```python
from build123d import *

# Parameters (mm, degrees)
SKETCH1_W           = 175
SKETCH1_H           = 77
SKETCH1_W_2         = 170
SKETCH1_H_2         = 69
BOSS_EXTRUDE1_DEPTH = 105
SKETCH2_W           = 175
SKETCH2_H           = 77
BOSS_EXTRUDE2_DEPTH = 3
SKETCH3_W           = 70
SKETCH3_H           = 80
SKETCH3_W_2         = 43
SKETCH3_H_2         = 62
CUT_EXTRUDE1_DEPTH  = 2.5
SKETCH4_W           = 12
SKETCH4_H           = 3
SKETCH4_W_2         = 24.903681778
SKETCH4_H_2         = 5
SKETCH4_W_3         = 25
SKETCH4_R           = 3
CUT_EXTRUDE2_DEPTH  = 12.5
SKETCH5_W           = 17.65
SKETCH5_H           = 18.35
CUT_EXTRUDE3_DEPTH  = 10
SKETCH6_W           = 5
SKETCH6_H           = 5
CUT_EXTRUDE4_DEPTH  = 10


with BuildPart() as part:
    # Sketch1 → Boss-Extrude1 (new body)
    with BuildSketch(Plane(origin=(0, 0, 0), x_dir=(1, 0, 0), z_dir=(0, 1, 0))):
        with Locations((-14.5, -36.5)):
            Rectangle(SKETCH1_W, SKETCH1_H)
        with Locations((-15, -35.5)):
            Rectangle(SKETCH1_W_2, SKETCH1_H_2, mode=Mode.SUBTRACT)
    extrude(amount=BOSS_EXTRUDE1_DEPTH)

    # Sketch2 → Boss-Extrude2 (add)
    with BuildSketch(Plane(origin=(0, 0, 0), x_dir=(-1, 0, 0), z_dir=(0, -1, 0))):
        with Locations((14.5, -36.5)):
            Rectangle(SKETCH2_W, SKETCH2_H)
    extrude(amount=-BOSS_EXTRUDE2_DEPTH)

    # Sketch3 → Cut-Extrude1 (cut)
    with BuildSketch(Plane.XY.offset(75)):
        with Locations((31, 57)):
            Rectangle(SKETCH3_W, SKETCH3_H)
        with Locations((-73.5, 66)):
            Rectangle(SKETCH3_W_2, SKETCH3_H_2)
    extrude(amount=-CUT_EXTRUDE1_DEPTH, mode=Mode.SUBTRACT)

    # Sketch4 → Cut-Extrude2 (cut)
    with BuildSketch(Plane.XY.offset(75)):
        with Locations((-28, 88.5)):
            Rectangle(SKETCH4_W, SKETCH4_H)
        with Locations((-73.5, 32.5)):
            Rectangle(SKETCH4_W_2, SKETCH4_H_2)
        with Locations((31, 14.5)):
            Rectangle(SKETCH4_W_3, SKETCH4_H_2)
        with Locations((-28, 51)):
            Circle(SKETCH4_R)
    extrude(amount=-CUT_EXTRUDE2_DEPTH, mode=Mode.SUBTRACT)

    # Sketch5 → Cut-Extrude3 (cut)
    with BuildSketch(Plane.XY.offset(1)):
        with Locations((48.75, 12.175)):
            Rectangle(SKETCH5_W, SKETCH5_H)
    extrude(amount=-CUT_EXTRUDE3_DEPTH, mode=Mode.SUBTRACT)

    # Sketch6 → Cut-Extrude4 (cut)
    with BuildSketch(Plane.ZY.offset(-70)):
        with Locations((35.5, 5.5)):
            Rectangle(SKETCH6_W, SKETCH6_H)
    extrude(amount=-CUT_EXTRUDE4_DEPTH, mode=Mode.SUBTRACT)


solid = part.part
```
CAD build for the part. Positions are in the model's coordinates, mm. A direction names the side the tool comes from. Coordinates: 2 decimals unless noted, no trailing zeros. Order: outer loops, then holes, each group sorted by start corner. A loop starts at its lowest first (then second) coordinate and runs counter-clockwise, first axis right, second up. Notation, with made-up numbers: (-8.5, 68.25) - (34.5, 68.25) arc R18 cw to (34.5, 100.25) - close; hole circle Ø2 at (43.25, -26). An arc over 180 degrees is marked (long way). Answer in a Markdown table with one row per item.
1. Drill centre lines: L1, parallel to Y at x = -28, z = 73.25; L2, parallel to Z at x = 40.5, y = 51; L3, parallel to X at y = 15, z = 70.5. Where is each one in solid material? Low to high. Write a range as from..to.
Answer:
| item | result |
|---|---|
| L1 | 0..48, 54..87, 90..105 |
| L2 | -2..1, 70..72.5 |
| L3 | -102..18.5, 43.5..73 |
2. Slice it at A-A, the plane y = 14. List the corners of the cut face in (x, z) (3 decimals).
Answer:
| item | result |
|---|---|
| outline | (-102, -2) - (39.925, -2) - (39.925, 1) - (-100, 1) - (-100, 70) - (18.5, 70) - (18.5, 75) - (-102, 75) - close; (43.5, 70) - (70, 70) - (70, 1) - (57.575, 1) - (57.575, -2) - (73, -2) - (73, 75) - (43.5, 75) - close |
3. Slice it at D-D, the plane x = -28. List the corners of the cut face in (y, z).
Answer:
| item | result |
|---|---|
| outline | (0, -2) - (105, -2) - (105, 1) - (3, 1) - (3, 70) - (48, 70) - (48, 75) - (0, 75) - close; (54, 70) - (87, 70) - (87, 75) - (54, 75) - close; (90, 70) - (105, 70) - (105, 75) - (90, 75) - close |
4. Pull direction Z, two halves, no side cores. Call faces 4 (the face through (-16, 52, -2)), 5 (the face through (-15, 3, 35)), 6 (the face through (43.5, 14, 73)): +Z half, -Z half, draft (parallel to the pull), parting line (faces both ways), or undercut.
Answer:
| item | result |
|---|---|
| face 4 | -Z half |
| face 5 | undercut |
| face 6 | draft |
5. 3-axis set-ups, long thin cutter, end or side, ignore diameter. For faces 1 (the face through (-28, 90, 73)), 2 (the face through (-16, 0, 36)), 3 (the face through (-16, 53, 70)): which of +Z, -Z, +X, -X, +Y, -Y reach the whole face in a straight line?
Answer:
| item | result |
|---|---|
| face 1 | +Z |
| face 2 | +Z, -Z, +X, -X, -Y |
| face 3 | +Y |
6. Slice it at B-B, the plane x = 49. List the corners of the cut face in (y, z).
Answer:
| item | result |
|---|---|
| outline | (0, -2) - (3, -2) - (3, 70) - (105, 70) - (105, 75) - (97, 75) - (97, 72.5) - (17, 72.5) - (17, 75) - (0, 75) - close; (21.35, -2) - (105, -2) - (105, 1) - (21.35, 1) - close |
7. Flat gauge pins, fed straight in: P1, Ø2, axis at x = -80.5, y = 94.5, coming from the +Z side; P2, Ø5, axis at x = -28, y = 51, coming from the +Z side; P3, Ø3, axis at x = -8.5, z = 62, coming from the +Y side. Where does each tip first touch, or does it go through?
Answer:
| item | result |
|---|---|
| P1 | z = 72.5 |
| P2 | z = 1 |
| P3 | y = 3 |
8. Slice it at C-C, the plane z = 26.5. List the corners of the cut face in (x, y).
Answer:
| item | result |
|---|---|
| outline | (-102, 0) - (73, 0) - (73, 105) - (70, 105) - (70, 3) - (-100, 3) - (-100, 105) - (-102, 105) - close |
